The model under review builds one solid part; all positions refer to its coordinate system, in mm. A direction names the side the tool comes from. Give positions to 0.01 mm unless a question says otherwise; leave off trailing zeros. Loops run counter-clockwise (first coordinate to the right, second up) from the corner with the lowest first, then second, coordinate; pieces in that order, holes last. Notation, with made-up numbers: M -31.75,56.25 L -8.75,56.25 A20 cw -8.75,90.25 Z; hole C -11.75,86 d7. An arc over 180 degrees is marked long. Put each result on its own line as item: value. Start each with the question number.
Autodesk Inventor part; units mm, degrees
ref_plane "YZ Plane" through (0, 0, 0) normal (1, 0, 0) x (0, 1, 0)
ref_plane "XZ Plane" through (0, 0, 0) normal (0, 1, 0) x (-1, 0, 0)
ref_plane "XY Plane" through (0, 0, 0) normal (0, 0, 1) x (1, 0, 0)
sketch "Sketch1" plane through (0, 0, 0) normal (0, 1, 0) x (-1, 0, 0)
  line L0 (0, -7.9375) -> (0, 7.9375) construction
  line L1 (17.4625, -7.9375) -> (17.4625, 7.9375) construction
  line L2 (-17.4625, 7.9375) -> (-17.4625, -7.9375) construction
  arc A0 (-17.4625, -7.9375) -> (17.4625, -7.9375) centre (0, -7.9375) ccw construction
  arc A1 (17.4625, 7.9375) -> (-17.4625, 7.9375) centre (0, 7.9375) ccw construction
  line L3 (14.1605, 7.9375) -> (14.1605, -7.9375)
  arc A2 (-14.1605, -7.9375) -> (14.1605, -7.9375) centre (0, -7.9375) ccw
  line L4 (-14.1605, -7.9375) -> (-14.1605, 7.9375)
  arc A3 (14.1605, 7.9375) -> (-14.1605, 7.9375) centre (0, 7.9375) ccw
  line L5 (10.9855, -7.9375) -> (10.9855, 7.9375)
  arc A4 (10.9855, 7.9375) -> (-10.9855, 7.9375) centre (0, 7.9375) ccw
  line L6 (-10.9855, 7.9375) -> (-10.9855, -7.9375)
  arc A5 (-10.9855, -7.9375) -> (10.9855, -7.9375) centre (0, -7.9375) ccw
  point P0 (0, 0)
  point P1 (0, 25.4)
  point P2 (0, -25.4)
  dimension "d1" = 34.925
  dimension "d2" = 3.302
  dimension "d3" = 50.8
  dimension "d15" = 3.175
extrude "Extrusion1" add sketch "Sketch1" along normal mid plane 25.4
chamfer "Chamfer2" distance 1.5875 angle 45 4 edges at (0, 12.7, 22.098) (14.1605, 12.7, 0) (0, 12.7, -22.098) (-14.1605, 12.7, 0)
properties part number "WL-006" material "Aluminum 6061"
(1) We need section B-B, the plane z = -4.5. Write out the cut boundary in (x, y), plus the area to 3 significant figures.
(2) To check wall thickness, follow L1, parallel to X at y = -6, z = 3; L2, parallel to X at y = -0.75, z = -18; L3, parallel to Z at x = 2, y = 0.5. State the ranges of each line that lie inside material, in increasing order. Write a range as [from, to].
(3) Insertion check: pin 1 (1 mm diameter, centred on x = 1, y = 1, fed in from -Z); pin 2 (2 mm diameter, centred on y = 3.5, z = 12.5, fed in from +X); pin 3 (5 mm diameter, centred on x = 7.5, y = 1.5, fed in from +Z). Each pin has a flat end and moves straight along its axis. Give the tip position at first contact, or say it passes through.
(4) We need section A-A, the plane x = 0. Write out the cut boundary in (y, z).
(5) Draft analysis for pull direction Z (two halves, no side actions). For faces 3 (the flat face through (-10.986, 0, 0)), 4 (the cylindrical face through (0.311, -0.96, 22.095)), 5 (the cylindrical face through (-0.311, -0.96, -22.095)), 6 (the flat face through (-14.16, -1, 0)), state which applies: +Z half, -Z half, draft (parallel to the pull), parting line (faces both ways), or undercut.
(6) For faces 1 (the cylindrical face through (-0.24, -0.18, -18.92)), 2 (the conical face through (0.283, 12.424, 20.783)), list the 3-axis set-ups (+Z, -Z, +X, -X, +Y, -Y) from which the entire face can be reached by the end or side of a thin tool; tool diameter is ignored.
(7) We need section C-C, the plane y = -9.5. Write out the cut boundary in (x, z), plus the area to 3 significant figures.
Check sheet entries:
1. outline: M -14.16,-12.7 L -10.99,-12.7 L -10.99,12.7 L -12.57,12.7 L -14.16,11.11 Z; M 10.99,-12.7 L 14.16,-12.7 L 14.16,11.11 L 12.57,12.7 L 10.99,12.7 Z
1. area: 159 mm²
2. L1: x = [-14.16, -10.99], [10.99, 14.16]
2. L2: x = [-9.96, -4.41], [4.41, 9.96]
2. L3: z = [-21.96, -18.74], [18.74, 21.96]
3. pin 1: stops at z = -22.09
3. pin 2: stops at x = 13.71
3. pin 3: stops at z = 21.19
4. outline: M -12.7,-22.1 L 11.11,-22.1 L 12.7,-20.51 L 12.7,-18.92 L -12.7,-18.92 Z; M -12.7,18.92 L 12.7,18.92 L 12.7,20.51 L 11.11,22.1 L -12.7,22.1 Z
5. face 3: undercut
5. face 4: +Z half
5. face 5: -Z half
5. face 6: draft
6. face 1: +Y, -Y
6. face 2: +Z, +Y
7. outline: M -14.16,-7.94 A14.16 ccw 14.16,-7.94 L 14.16,7.94 A14.16 ccw -14.16,7.94 Z; hole M -10.99,-7.94 A10.99 ccw 10.99,-7.94 L 10.99,7.94 A10.99 ccw -10.99,7.94 Z
7. area: 352 mm²
